The listing builds one solid part. Answer for the finished solid, in the listing's coordinates (mm). Round coordinates to 2 decimals unless told otherwise and drop trailing zeros. Loops run counter-clockwise (first coordinate to the right, second up) from the corner with the lowest first, then second, coordinate; pieces in that order, holes last. Notation, with made-up numbers: (46, 4.5) -> (93, 4.5) arc R28 cw to (93, 37.5) -> close; hole circle Ø6 at (87, 84). An arc over 180 degrees is marked (long way). Write each question's results on one line, items separated by ' | '. Start each with the question number.
(1) Straight lines are drawn through the part: probe 1 along Z at (x, y) = (0, -0.55); probe 2 along X at (y, z) = (1.05, -59.1); probe 3 along Z at (x, y) = (0.5, 1.85). For each, find the intervals that lie inside material, in ascending order.
(2) The part is cut by section A-A (z = -59.1). Determine the outline of the cut face in (x, y), plus the area to 3 significant figures.
(3) The part is cut by section C-C (y = 1.65). Count the separate pieces of the cut face and the enclosed holes in it, plus the area to 3 significant figures.
(4) A flat-ended cylindrical pin translates along its axis: pin 1 (2 mm diameter, centred on x = 0, z = -59.1, fed in from -Y). Find the tip coordinate at first contact, or state that the pin passes through.
(5) The part is cut by section B-B (z = -12.5). Determine the outline of the cut face in (x, y), plus the area to 3 significant figures.
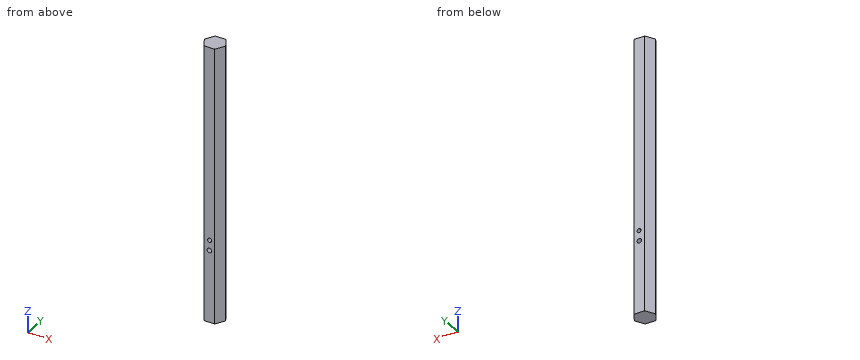
Autodesk Inventor part; units mm, degrees
ref_plane "YZ Plane" through (0, 0, 0) normal (1, 0, 0) x (0, 1, 0)
ref_plane "XZ Plane" through (0, 0, 0) normal (0, 1, 0) x (-1, 0, 0)
ref_plane "XY Plane" through (0, 0, 0) normal (0, 0, 1) x (1, 0, 0)
sketch "Sketch1" plane through (0, 0, 0) normal (0, 0, 1) x (1, 0, 0)
  line L0 (0, 0) -> (3.1, 0) construction
  circle A0 centre (0, 0) radius 7.5
  line L1 (0, 0) -> (1.55, 2.6847) construction
  line L2 (0, 0) -> (-1.55, 2.6847) construction
  line L3 (0, 0) -> (-3.1, 0) construction
  line L4 (0, 0) -> (-1.55, -2.6847) construction
  line L5 (0, 0) -> (1.55, -2.6847) construction
  line L6 (-1.55, 2.6847) -> (1.55, 2.6847)
  line L7 (1.55, 2.6847) -> (3.1, 0)
  line L8 (3.1, 0) -> (1.55, -2.6847)
  line L9 (1.55, -2.6847) -> (-1.55, -2.6847)
  line L10 (-1.55, -2.6847) -> (-3.1, 0)
  line L11 (-3.1, 0) -> (-1.55, 2.6847)
  line L12 (-1.7809, 3.0847) -> (1.7809, 3.0847)
  dimension "d0" = 3.1
  dimension "d3" = 360
extrude "Extrusion1" add sketch "Sketch1" against normal blind 80 contours L6 L7 L8 L9 L10 L11
sketch "Sketch2" plane through (-1.55, -2.6847, 0) normal (0, -1, 0) x (1, 0, 0)
  line L0 (0, 0) -> (0, -80)
  line L1 (3.1, 0) -> (3.1, -80)
  line L2 (106.9037, -80.1) -> (-63.0931, -80.1)
  ellipse E0 centre (1.709, -56.1) end of major axis (1.709, -55.45) minor radius 0.65
  line L3 (1.709, -56.1) -> (-0.1699, -56.1) construction
  circle A0 centre (1.55, -56.1) radius 0.65
  line L4 (0, 0) -> (3.1, 0)
  circle A1 centre (1.55, -59.1) radius 0.65
  point P0 (1.55, 0)
  point P1 (1.55, 0)
  point P2 (1.6295, -55.4549)
  point P3 (1.6295, -56.7451)
  dimension "d7" = 1.3
  dimension "d8" = 56.1
  dimension "d9" = 3
extrude "Extrusion2" cut sketch "Sketch2" against normal blind 10 contours E0 A0 | A1 picked at (1.8134, -56.0482)
properties part number "eje2_n"
Checked values:
1) probe 1: z = -80 to -59.75, -58.45 to -56.73, -55.47 to 0 | probe 2: x = -2.49 to -0.65, 0.65 to 2.49 | probe 3: z = -80 to -59.52, -58.68 to -56.52, -55.68 to 0
2) outline: (-3.1, 0) -> (-1.55, -2.68) -> (-0.65, -2.68) -> (-0.65, 2.68) -> (-1.55, 2.68) -> close; (0.65, -2.68) -> (1.55, -2.68) -> (3.1, 0) -> (1.55, 2.68) -> (0.65, 2.68) -> close | area: 18.0 mm2
3) separate pieces: 1 | enclosed holes: 2 | area: 341 mm2
4) pin 1: stops at y = -2.68
5) outline: (-3.1, 0) -> (-1.55, -2.68) -> (1.55, -2.68) -> (3.1, 0) -> (1.55, 2.68) -> (-1.55, 2.68) -> close | area: 25.0 mm2
